Input: part model. Units: mm. Frame: model coordinates. Face numbers are marked on the shaded views. A direction names the side the tool comes from. Round coordinates to 2 decimals unless told otherwise and drop trailing zeros. Loops run counter-clockwise (first coordinate to the right, second up) from the corner with the lowest first, then second, coordinate; pieces in that order, holes last. Notation, with made-up numbers: M -34,-5 L 20,-5 A32 cw 20,29 Z; hole C 39,30.5 d10. An arc over 180 degrees is marked long. Put each result on its own line as item: value. Start each with the question number.
1) Draft query along Y for the marked faces 1, 2 and 3. Return one class per face: +Y half, -Y half, draft (parallel to the pull), parting line (faces both ways), or undercut.
2) Reachability of the marked faces 4 and 5 from +Z, -Z, +X, -X, +Y, -Y: full face, straight path, thin tool, end or side. Return the list, or none.
3) Section B-B on x = -511.65. Output: boundary loops of the cut face in (y, z) (3 decimals), plus the area to 3 significant figures.
4) Section A-A on z = 0. Output: boundary loops of the cut face in (x, y) (3 decimals), plus the area to 3 significant figures.
5) Line query: probe 1 along Z at (x, y) = (-494, 5.5); probe 2 along Y at (x, z) = (-517.5, 1.5) (3 decimals); probe 3 along X at (y, z) = (20.75, -0.5). Output: solid intervals per line, ascending.
6) Pin query (flat end, axial travel): pin 1 (8 mm diameter, centred on x = -489.5, z = 2.5, fed in from +Y); pin 2 (6 mm diameter, centred on y = 13, z = 5, fed in from -X); pin 3 (1 mm diameter, centred on x = -511, z = 4.5, fed in from -Y) (3 decimals); pin 4 (10 mm diameter, centred on y = 21, z = -0.5, fed in from +X). Return the tip coordinate at first contact, or that it passes through.
7) Section C-C on x = -479. Output: boundary loops of the cut face in (y, z).
8) Section D-D on z = -7. Output: boundary loops of the cut face in (x, y) (3 decimals), plus the area to 3 significant figures.
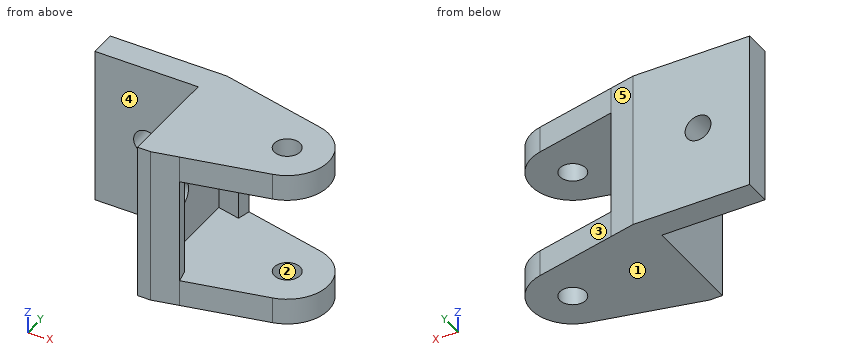
Autodesk Inventor part; units mm, degrees
ref_plane "YZ Plane" through (0, 0, 0) normal (1, 0, 0) x (0, 1, 0)
ref_plane "XZ Plane" through (0, 0, 0) normal (0, 1, 0) x (-1, 0, 0)
ref_plane "XY Plane" through (0, 0, 0) normal (0, 0, 1) x (1, 0, 0)
ref_plane "Work Plane1" through (0, 0, 0) normal (0, 0, 1) x (1, 0, 0)
sketch "Sketch1" plane through (0, 0, 0) normal (0, 0, 1) x (1, 0, 0)
  line L0 (-521.65, -0.245) -> (-521.65, -0.245)
  line L1 (-521.65, 19.755) -> (-521.65, -0.245)
  line L2 (-521.65, 19.755) -> (-521.65, 19.755)
  line L3 (-521.65, -0.245) -> (-521.65, 19.755)
  line L4 (-501.65, 19.755) -> (-501.65, 19.755)
  line L5 (-501.65, -0.245) -> (-501.65, 19.755)
  line L6 (-501.65, -0.245) -> (-501.65, -0.245)
  line L7 (-501.65, 19.755) -> (-501.65, -0.245)
  line L8 (-521.65, -0.245) -> (-521.65, -0.245)
  line L9 (-521.65, 19.755) -> (-521.65, -0.245)
  line L10 (-521.65, 19.755) -> (-521.65, 19.755)
  line L11 (-521.65, -0.245) -> (-521.65, 19.755)
  line L12 (-501.65, 19.755) -> (-499.11, 19.755)
  line L13 (-499.11, 19.755) -> (-499.11, -0.245)
  line L14 (-499.11, -0.245) -> (-501.65, -0.245)
  line L15 (-501.65, -0.245) -> (-501.65, 19.755)
  line L16 (-499.11, 19.755) -> (-521.65, 19.755)
  line L17 (-521.65, 19.755) -> (-521.65, 24.835)
  line L18 (-521.65, 24.835) -> (-499.11, 24.835)
  line L19 (-499.11, 24.835) -> (-499.11, 19.755)
  point P0 (0, 0)
  dimension "d0" = 2.54
  dimension "d1" = 5.08
extrude "Extrusion1" add sketch "Sketch1" along normal mid plane 30.48
sketch "Sketch2" plane through (-521.65, 24.835, 15.24) normal (0, 1, 0) x (1, 0, 0)
  line L0 (0, 30.48) -> (0, 0)
  line L1 (22.54, 0) -> (0, 0)
  line L2 (22.54, 30.48) -> (22.54, 0)
  line L3 (0, 30.48) -> (22.54, 30.48)
  line L4 (20, 345.44) -> (20, -314.96)
  line L5 (0, 30.48) -> (0, 0)
  line L6 (0, 15.24) -> (20, 15.24)
  circle A0 centre (10, 15.24) radius 2.5
  point P0 (521.65, 15.24)
  dimension "d4" = 5
extrude "Extrusion2" cut sketch "Sketch2" against normal blind 25.4 contours A0 L6 | L6 A0
sketch "Sketch3" plane through (-501.65, -0.245, 15.24) normal (-1, 0, 0) x (0, 0, 1)
  line L0 (-345.44, 0) -> (314.96, 0)
  line L1 (-30.48, 20) -> (0, 20)
  line L2 (-15.24, 20) -> (-15.24, 0)
  line L3 (-30.48, 0) -> (0, 0)
  circle A0 centre (-15.24, 10) radius 2.5
  point P0 (-15.24, 0.245)
  dimension "d7" = 5
extrude "Extrusion3" cut sketch "Sketch3" against normal blind 25.4
sketch "Sketch4" plane through (0, 0, -15.24) normal (0, 0, -1) x (-1, 0, 0)
  line L0 (499.11, -0.245) -> (499.11, 24.835)
  line L1 (499.11, 24.835) -> (499.11, -0.245)
  line L2 (499.11, 12.295) -> (480.06, 12.295)
  line L3 (499.11, 12.295) -> (518.16, 12.295) construction
  arc A0 (478.2847, 20.0955) -> (478.2847, 4.4944) centre (480.06, 12.295) ccw
  circle A1 centre (480.06, 12.295) radius 2.5
  line L4 (499.11, 24.835) -> (478.2847, 20.0955)
  line L5 (499.11, -0.245) -> (478.2847, 4.4944)
  point P0 (0, 0)
  dimension "d10" = 19.05
  dimension "d11" = 180
  dimension "d12" = 16
  dimension "d13" = 5
extrude "Extrusion4" add sketch "Sketch4" against normal blind 5.08
sketch "Sketch5" plane through (0, 0, 15.24) normal (0, 0, 1) x (1, 0, 0)
  circle A0 centre (-480.06, 12.295) radius 2.5
  line L0 (-499.11, -0.245) -> (-499.11, 24.835)
  line L1 (-499.11, -0.245) -> (-478.2847, 4.4944)
  arc A1 (-478.2847, 4.4944) -> (-478.2847, 20.0955) centre (-480.06, 12.295) ccw
  line L2 (-478.2847, 20.0955) -> (-499.11, 24.835)
  point P0 (0, 0)
extrude "Extrusion5" add sketch "Sketch5" against normal blind 5.08
sketch "Sketch6" plane through (-499.11, -0.245, 10.16) normal (0.2219, -0.9751, 0) x (0.9751, 0.2219, 0)
  line L0 (0, 5.08) -> (21.3578, 5.08)
  line L1 (0, 0) -> (0, 5.08)
  line L2 (21.3578, 0) -> (0, 0)
  line L3 (21.3578, 5.08) -> (21.3578, 0)
  line L4 (21.3578, -25.4) -> (0, -25.4)
  line L5 (21.3578, -25.4) -> (21.3578, -20.32)
  line L6 (0, -20.32) -> (21.3578, -20.32)
  line L7 (0, -25.4) -> (0, -20.32)
  line L8 (0, -20.32) -> (0, 0)
  line L9 (21.3578, -25.4) -> (0, -25.4)
  line L10 (0, 5.08) -> (5.08, 5.08)
  line L11 (5.08, 5.08) -> (5.08, -25.4)
  line L12 (5.08, -25.4) -> (0, -25.4)
  line L13 (0, -25.4) -> (0, 5.08)
  point P0 (486.7204, -10.16)
  dimension "d18" = 5.08
extrude "Extrusion6" add sketch "Sketch6" against normal blind 2.54 contours L0 L11 L2 L1 | L2 L11 L6 L8 | L6 L11 L4 L7
sketch "Sketch7" plane through (-499.11, 24.835, -10.16) normal (0.2219, 0.9751, 0) x (0.9751, -0.2219, 0)
  line L0 (21.3578, -25.4) -> (0, -25.4)
  line L1 (21.3578, -25.4) -> (21.3578, -20.32)
  line L2 (0, -20.32) -> (21.3578, -20.32)
  line L3 (0, -20.32) -> (0, -25.4)
  line L4 (0, 5.08) -> (21.3578, 5.08)
  line L5 (0, 5.08) -> (0, 0)
  line L6 (21.3578, 0) -> (0, 0)
  line L7 (21.3578, 5.08) -> (21.3578, 0)
  line L8 (0, -25.4) -> (5.08, -25.4)
  line L9 (5.08, -25.4) -> (5.08, 5.08)
  line L10 (5.08, 5.08) -> (0, 5.08)
  line L11 (0, 5.08) -> (0, -25.4)
  point P0 (492.1771, -10.16)
  dimension "d21" = 5.08
extrude "Extrusion7" add sketch "Sketch7" against normal blind 2.54 contours L0 L3 L2 L9 | L2 L11 L6 L9 | L6 L5 L4 L9
properties part number "YIdler"
Geometry results:
1. face 1: draft
1. face 2: undercut
1. face 3: +Y half
2. face 4: +Z, -Z, -X, -Y
2. face 5: +Z, -Z, +X, +Y
3. outline: M 19.755,-15.24 L 24.835,-15.24 L 24.835,-2.5 L 19.755,-2.5 Z; M 19.755,2.5 L 24.835,2.5 L 24.835,15.24 L 19.755,15.24 Z
3. area: 129 mm²
4. outline: M -521.65,19.755 L -514.15,19.755 L -514.15,24.835 L -521.65,24.835 Z; M -509.15,19.755 L -501.65,19.755 L -501.65,12.255 L -499.11,12.255 L -499.11,22.23 L -494.72,21.231 L -494.157,23.708 L -499.11,24.835 L -509.15,24.835 Z; M -501.65,-0.245 L -499.11,-0.245 L -494.157,0.882 L -494.72,3.359 L -499.11,2.36 L -499.11,7.255 L -501.65,7.255 Z
4. area: 152 mm²
5. probe 1: z = -15.24 to -10.16, 10.16 to 15.24
5. probe 2: y = 19.755 to 24.835
5. probe 3: x = -521.65 to -514.1, -509.2 to -499.11
6. pin 1: passes through
6. pin 2: stops at x = -501.65
6. pin 3: stops at y = 19.755
6. pin 4: stops at x = -494.16
7. outline: M 4.33,-15.24 L 10.03,-15.24 L 10.03,-10.16 L 4.33,-10.16 Z; M 4.33,10.16 L 10.03,10.16 L 10.03,15.24 L 4.33,15.24 Z; M 14.56,-15.24 L 20.26,-15.24 L 20.26,-10.16 L 14.56,-10.16 Z; M 14.56,10.16 L 20.26,10.16 L 20.26,15.24 L 14.56,15.24 Z
8. outline: M -521.65,19.755 L -501.65,19.755 L -501.65,-0.245 L -499.11,-0.245 L -494.157,0.882 L -494.72,3.359 L -499.11,2.36 L -499.11,22.23 L -494.72,21.231 L -494.157,23.708 L -499.11,24.835 L -521.65,24.835 Z
8. area: 190 mm²
